Work out the finished part from the listing and answer in its coordinate system (mm). A direction names the side the tool comes from. Coordinates: 2 decimals unless noted, no trailing zeros. Write each loop counter-clockwise with the first axis right and the second up, starting at its lowest first coordinate (ties: lowest second). Pieces come first, ordered by that corner, then holes. Notation, with made-up numbers: (46, -31.5) - (105, -31.5) arc R18 ccw to (105, -15.5) - close; hole circle Ø2 at (8.5, -1.75). An arc over 180 degrees is marked (long way). Use a Markdown table: item, result. Add a question column.
(1) The part is cut by section D-D, the plane z = 64. Give the vertices of the cut face in (x, y) (1 decimal).
(2) Find the intervals of material crossed by line 1 (X direction, y = 0, z = 618); line 2 (X direction, y = -5.5, z = 625.5), in increasing order. Write a range as from..to.
(3) A tool of negligible diameter and unlimited length cuts with its end or side. For faces 1 (the face through (0, 37, 508)), 2 (the face through (31, -20, 662.94)), from which of +Z, -Z, +X, -X, +Y, -Y can it reach the whole face along a straight path? Write none if from no direction.
(4) The part is cut by section C-C, the plane y = 21.5. Give the vertices of the cut face in (x, z), then the cut area to 3 significant figures.
(5) The part is cut by section B-B, the plane y = -31. Give the vertices of the cut face in (x, z).
(6) The part is cut by section A-A, the plane x = 0. Give the vertices of the cut face in (y, z), then the cut area to 3 significant figures.
(7) Given pin 1 Ø12 at (y, z) = (-20.5, 492.5) entering from +X; pin 2 Ø2 at (x, z) = (-1.5, 169) entering from -Y; pin 3 Ø1.5 at (x, z) = (14.5, 353) entering from -Y; pin 4 Ø19 at (x, y) = (0, 22.5) entering from +Z, each flat-ended and moving along its own axis, determine where each tip first touches the part or whether it passes through.
from build123d import *

# Parameters (mm, degrees)
SKETCH1_R           = 38.0746
SKETCH1_R_2         = 36.5125
BOSS_EXTRUDE1_DEPTH = 76.2
BOSS_EXTRUDE2_DEPTH = 431.8
SKETCH3_R           = 38.0746
SKETCH3_R_2         = 36.5125
BOSS_EXTRUDE3_DEPTH = 154.94


with BuildPart() as part:
    # Sketch1 → Boss-Extrude1 (new body)
    with BuildSketch(Plane.XY):
        with Locations(Location((0, 0, 0), (0, 0, 180))):
            Circle(SKETCH1_R)
        with Locations(Location((0, 0, 0), (0, 0, 180))):
            Circle(SKETCH1_R_2, mode=Mode.SUBTRACT)
    extrude(amount=BOSS_EXTRUDE1_DEPTH)

    # Sketch2 → Boss-Extrude2 (add)
    with BuildSketch(Plane.XY.offset(76.2)):
        with BuildLine():
            Line((-38.0746, 0), (-36.5125, 0))
            ThreePointArc((-36.5125, 0), (0, -36.5125), (36.5125, 0))
            Line((36.5125, 0), (38.0746, 0))
            ThreePointArc((38.0746, 0), (0, -38.0746), (-38.0746, 0))
        make_face()
    extrude(amount=BOSS_EXTRUDE2_DEPTH)

    # Sketch3 → Boss-Extrude3 (add)
    with BuildSketch(Plane.XY.offset(508)):
        Circle(SKETCH3_R)
        Circle(SKETCH3_R_2, mode=Mode.SUBTRACT)
    extrude(amount=BOSS_EXTRUDE3_DEPTH)


solid = part.part
Model answer:
| question | item | result |
|---|---|---|
| 1 | outline | circle Ø76.1 at (0, 0); hole circle Ø73 at (0, 0) |
| 2 | line 1 | -38.07..-36.51, 36.51..38.07 |
| 2 | line 2 | -37.68..-36.1, 36.1..37.68 |
| 3 | face 1 | +X, -X, +Y |
| 3 | face 2 | +Z, +X, -X, +Y, -Y |
| 4 | outline | (-31.42, 0) - (-29.51, 0) - (-29.51, 76.2) - (-31.42, 76.2) - close; (-31.42, 508) - (-29.51, 508) - (-29.51, 662.94) - (-31.42, 662.94) - close; (29.51, 0) - (31.42, 0) - (31.42, 76.2) - (29.51, 76.2) - close; (29.51, 508) - (31.42, 508) - (31.42, 662.94) - (29.51, 662.94) - close |
| 4 | area | 884 mm^2 |
| 5 | outline | (-22.11, 0) - (-19.29, 0) - (-19.29, 662.94) - (-22.11, 662.94) - close; (19.29, 0) - (22.11, 0) - (22.11, 662.94) - (19.29, 662.94) - close |
| 6 | outline | (-38.07, 0) - (-36.51, 0) - (-36.51, 662.94) - (-38.07, 662.94) - close; (36.51, 0) - (38.07, 0) - (38.07, 76.2) - (36.51, 76.2) - close; (36.51, 508) - (38.07, 508) - (38.07, 662.94) - (36.51, 662.94) - close |
| 6 | area | 1,400 mm^2 |
| 7 | pin 1 | x = 35.21 |
| 7 | pin 2 | y = -38.07 |
| 7 | pin 3 | y = -35.51 |
| 7 | pin 4 | through |
